Check sheet for the modelled part. Datum: model origin and axes. Units: mm. A direction names the side the tool comes from. Coordinates: 2 decimals unless noted, no trailing zeros. Loops run counter-clockwise (first coordinate to the right, second up) from the corner with the lowest first, then second, coordinate; pieces in that order, holes last. Notation, with made-up numbers: (69.25, -33.75) -> (97.25, -33.75) arc R17 cw to (97.25, -13.75) -> close; hole circle Ø10 at (15.25, 75). An arc over 180 degrees is marked (long way). Use CSV: the item, a comma, the result in double quotes.
```python
from build123d import *

# Parameters (mm, degrees)
LPATTERN1_COUNT       = 11
LPATTERN1_PITCH       = 3
SKETCH3_R             = 5.000000000000004
BOSS_EXTRUDE1_DEPTH   = 3
SKETCH4_R             = 1.75
CUT_EXTRUDE1_DEPTH    = 43.81938813201328
CHAMFER1_SIZE         = 2
SKETCH5_R             = 1.2499999999999991
SKETCH5_R_2           = 1.2500000000000002
CUT_EXTRUDE2_DEPTH    = 2
SKETCH6_R             = 12.499999999999995
CUT_EXTRUDE3_DEPTH    = 1
CUT_EXTRUDE5_REACH    = 37.686
SKETCH7_R             = 12.499999999999996
SKETCH7_R_2           = 3.4999999999999982
SKETCH8_R             = 4.999999999999997
SKETCH8_R_2           = 3.4999999999999982
BOSS_EXTRUDE2_DEPTH   = 8
BOSS_EXTRUDE3_START   = 0.5
SKETCH9_R             = 12.499999999999996
SKETCH9_R_2           = 1.2499999999999991
SKETCH9_R_3           = 3.499999999999998
SKETCH9_R_4           = 1.2500000000000009
SKETCH9_R_5           = 1.2500000000000002
BOSS_EXTRUDE3_DEPTH   = 0.5
CROQUIS1_R            = 1.550000000000001
CORTAR_EXTRUIR1_DEPTH = 2.5


with BuildPart() as part:
    # Sketch1 → Revolve1 (revolve)
    with BuildSketch(Plane.XY, mode=Mode.PRIVATE) as revolve1_sk:
        Polygon((-2.5, -3.1e-16), (-2.5, 7.999999999999998), (-0.7999999999999999, 7.999999999999998), (-0.8, 36), (-12.5, 36), (-12.499999999999995, 0), align=None)
    revolve(revolve1_sk.sketch.rotate(Axis((0, 0, 0), (0, 1, 0)), 270), axis=Axis((0, 0, 0), (0, 1, 0)))

    # Sketch2 → Cut-Revolve1 (revolve, cut)
    with BuildSketch(Plane(origin=(0, 0, 0), x_dir=(0, 0, -1), z_dir=(1, 0, 0))):
        Polygon((12.499999999999996, 33.99999999999999), (3.4999999999999973, 33.99999999999999), (3.499999999999998, 31.999999999999993), (12.499999999999996, 31.999999999999993), align=None)
    cut_revolve1 = revolve(axis=Axis((0, 36, 0), (0, -1, 0)), mode=Mode.SUBTRACT)

    # LPattern1: Cut-Revolve1 ×11
    with Locations(*[(0, -i * LPATTERN1_PITCH, 0) for i in range(1, LPATTERN1_COUNT)]):
        add(cut_revolve1, mode=Mode.SUBTRACT)

    # Sketch3 → Boss-Extrude1 (add)
    with BuildSketch(Plane(origin=(0, 36, 0), x_dir=(1, 0, 0), z_dir=(0, 1, 0))):
        with Locations(Location((0, 0, 0), (0, 0, 90))):
            Circle(SKETCH3_R)
    extrude(amount=BOSS_EXTRUDE1_DEPTH)

    # Sketch4 → Cut-Extrude1 (cut, through all)
    with BuildSketch(Plane(origin=(0, 39, 0), x_dir=(1, 0, 0), z_dir=(0, 1, 0))):
        with Locations(Location((0, 0, 0), (0, 0, 270))):
            Circle(SKETCH4_R)
    extrude(amount=-CUT_EXTRUDE1_DEPTH, mode=Mode.SUBTRACT)

    # Chamfer1
    chamfer1_edges = [part.edges().sort_by_distance(p)[0] for p in [
        (5.4e-16, 39, -1.75),
    ]]
    chamfer(chamfer1_edges, length=CHAMFER1_SIZE)

    # Sketch5 → Cut-Extrude2 (cut)
    with BuildSketch(Plane(origin=(0, 36, 0), x_dir=(1, 0, 0), z_dir=(0, 1, 0))):
        with Locations(Location((9, -9.8e-16, 0), (0, 0, 270))):
            Circle(SKETCH5_R)
        with Locations(Location((-4.499999999999999, -7.794228634059948, 0), (0, 0, 270))):
            Circle(SKETCH5_R_2)
        with Locations(Location((-4.5000000000000036, 7.794228634059946, 0), (0, 0, 270))):
            Circle(SKETCH5_R_2)
    extrude(amount=-CUT_EXTRUDE2_DEPTH, mode=Mode.SUBTRACT)

    # Sketch6 → Cut-Extrude3 (cut)
    with BuildSketch(Plane.XZ):
        with Locations(Location((0, 0, 0), (0, 0, 270))):
            Circle(SKETCH6_R)
    extrude(amount=-CUT_EXTRUDE3_DEPTH, mode=Mode.SUBTRACT)

    # Sketch7 → Cut-Extrude5 (cut, up to next)
    with BuildSketch(Plane(origin=(0, 31.999999999999993, 0), x_dir=(1, 0, 0), z_dir=(0, 1, 0)), mode=Mode.PRIVATE) as cut_extrude5_sk1:
        with Locations(Location((0, 0, 0), (0, 0, 90))):
            Circle(SKETCH7_R)
        with Locations(Location((0, 0, 0), (0, 0, 270))):
            Circle(SKETCH7_R_2, mode=Mode.SUBTRACT)
    cut_extrude5_tool1 = extrude(cut_extrude5_sk1.sketch, amount=-CUT_EXTRUDE5_REACH, mode=Mode.PRIVATE) & part.part
    add(cut_extrude5_tool1.solids().sort_by_distance((0, 32, 12.146447))[0], mode=Mode.SUBTRACT)

    # Sketch8 → Boss-Extrude2 (add)
    with BuildSketch(Plane(origin=(0, 1.999999999999995, 0), x_dir=(1, 0, 0), z_dir=(0, 1, 0))):
        with Locations(Location((0, 0, 0), (0, 0, 90))):
            Circle(SKETCH8_R)
        with Locations(Location((0, 0, 0), (0, 0, 270))):
            Circle(SKETCH8_R_2, mode=Mode.SUBTRACT)
    extrude(amount=BOSS_EXTRUDE2_DEPTH)

    # Sketch9 → Boss-Extrude3 (add)
    with BuildSketch(Plane.XZ.offset(-33.99999999999999).offset(BOSS_EXTRUDE3_START)):
        with Locations(Location((0, 0, 0), (0, 0, 270))):
            Circle(SKETCH9_R)
        with Locations(Location((9, 9.8e-16, 0), (0, 0, 90))):
            Circle(SKETCH9_R_2, mode=Mode.SUBTRACT)
        with Locations(Location((0, 0, 0), (0, 0, 90))):
            Circle(SKETCH9_R_3, mode=Mode.SUBTRACT)
        with Locations(Location((-4.499999999999999, 7.794228634059948, 0), (0, 0, 90))):
            Circle(SKETCH9_R_4, mode=Mode.SUBTRACT)
        with Locations(Location((-4.5000000000000036, -7.794228634059946, 0), (0, 0, 90))):
            Circle(SKETCH9_R_5, mode=Mode.SUBTRACT)
    extrude(amount=-BOSS_EXTRUDE3_DEPTH)

    # Croquis1 → Cortar-Extruir1 (cut)
    with BuildSketch(Plane(origin=(0, 36, 0), x_dir=(1, 0, 0), z_dir=(0, 1, 0))):
        with Locations(Location((4.49999999999998, 7.7942286340599605, 0), (0, 0, 270))):
            Circle(CROQUIS1_R)
    extrude(amount=-CORTAR_EXTRUIR1_DEPTH, mode=Mode.SUBTRACT)


solid = part.part
```
1) Go/stop test with flat-tipped pins: pin 1 Ø1.5 at (x, z) = (-4.5, -7.79) entering from +Y; pin 2 Ø10 at (y, z) = (12.5, -9.5) entering from +X; pin 3 Ø1 at (x, z) = (-8.5, 3) entering from +Y; pin 4 Ø2 at (x, z) = (0.5, 0.5) entering from +Y. Record where each tip stops, or that it passes through.
Answer below:
pin 1,"stops at y = 29"
pin 2,"stops at x = 11.65"
pin 3,"stops at y = 36"
pin 4,"passes through"
2) Cross-section at B-B on y = 9. Record the boundary of the cut face in (x, z), and give its area (3 significant figures).
Answer below:
outline,"circle Ø10 at (0, 0); hole circle Ø3.5 at (0, 0)"
area,"68.9 mm²"
3) Access from +Z, -Z, +X, -X, +Y, -Y to the whole of each face (thin tool, end or side, straight path). Record for faces 1 (the cylindrical face through (-3.755, 25.493, -11.923)), 2 (the cylindrical face through (2.365, 26.986, 2.58)), 3 (the cylindrical face through (3.91, 34.77, -6.36)).
Answer below:
face 1,"+Y, -Y"
face 2,"none"
face 3,"+Y"
4) Thickness scan on line 1 along X through (y, z) = (34.5, 0); line 2 along Z through (x, y) = (4.5, 35.4); line 3 along X through (y, z) = (32, -1). Record the ranges inside material, lowest first. Write a range as from..to.
Answer below:
line 1,"x = -12.5..-1.75, 1.75..7.75, 10.25..12.5"
line 2,"z = -11.66..-9.34, -6.24..11.66"
line 3,"x = -3.35..-1.44, 1.44..3.35"
5) Draft check along Z on faces 4 (the cylindrical face through (-3.755, 4.493, -11.923)), 5 (the cylindrical face through (-4.02, 34.73, -6.64)), 6 (the flat face through (-3, 13, -3)). Enter one of: released by +Z, released by -Z, zero draft, split by the parting line, or undercut.
Answer below:
face 4,"split by the parting line"
face 5,"undercut"
face 6,"zero draft"
6) Cross-section at A-A on z = 0. Give the number of separate pieces and of enclosed holes in the cut face, and give its area (3 significant figures).
Answer below:
separate pieces,"3"
enclosed holes,"0"
area,"364 mm²"
